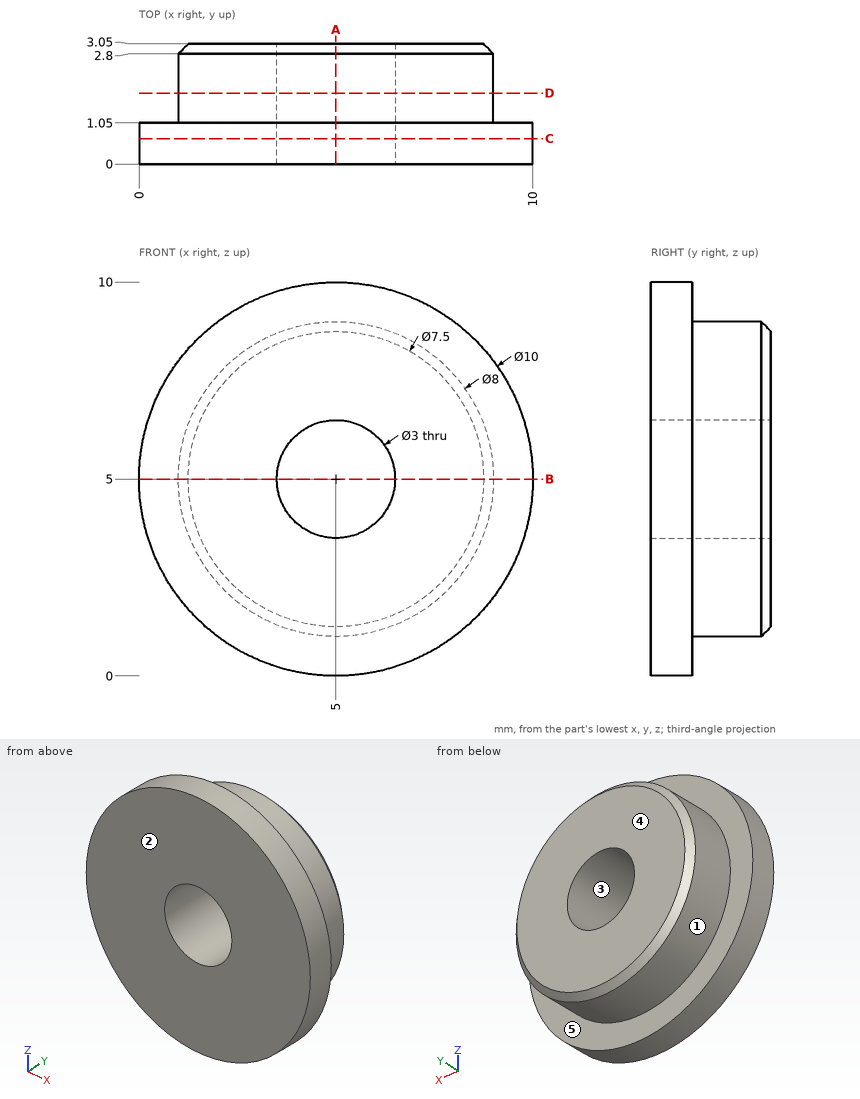
Geometry check sheet. Reference: drawing and pictorial views, mm from the part's lowest x, y, z. A direction names the side the tool comes from. Give positions to 0.01 mm unless a question says otherwise; leave off trailing zeros. Write each loop counter-clockwise with the first axis right and the second up, starting at its lowest first coordinate (ties: lowest second). Pieces come first, ordered by that corner, then holes.
Item 1: Cross-section at B-B (z = 5). Enter the section's corners in (x, y), and give its area (3 significant figures).
Item 2: Access from +Z, -Z, +X, -X, +Y, -Y to the whole of each face (thin tool, end or side, straight path). Record for the marked faces 4 and 5.
Item 3: Gauge pin test, flat end, axial feed: pin 1 (1.5 mm diameter, centred on y = 2.5, z = 5.5, fed in from -X). Record the tip position at first contact, or that the pin passes through.
Item 4: Scan lines: L1, parallel to X at y = 0.7, z = 5; L2, parallel to Z at x = 5, y = 1.9. Record each from-to range of solid material in increasing order.
Item 5: Cross-section at A-A (x = 5). Enter the section's corners in (y, z).
Item 6: Cross-section at D-D (y = 1.8). Enter the section's corners in (x, z).
Item 7: Draft check along Z on the marked faces 1, 2 and 3. Enter one of: released by +Z, released by -Z, zero draft, split by the parting line, or undercut.
Item 8: Cross-section at C-C (y = 0.65). Enter the section's corners in (x, z), and give its area (3 significant figures).
Report:
1. outline: (0, 0) - (3.5, 0) - (3.5, 3.05) - (1.25, 3.05) - (1, 2.8) - (1, 1.05) - (0, 1.05) - close; (6.5, 0) - (10, 0) - (10, 1.05) - (9, 1.05) - (9, 2.8) - (8.75, 3.05) - (6.5, 3.05) - close
1. area: 17.3 mm2
2. face 4: +Z, -Z, +X, -X, +Y
2. face 5: +Y
3. pin 1: stops at x = 1
4. L1: x = 0 to 3.5, 6.5 to 10
4. L2: z = 1 to 3.5, 6.5 to 9
5. outline: (0, 0) - (1.05, 0) - (1.05, 1) - (2.8, 1) - (3.05, 1.25) - (3.05, 3.5) - (0, 3.5) - close; (0, 6.5) - (3.05, 6.5) - (3.05, 8.75) - (2.8, 9) - (1.05, 9) - (1.05, 10) - (0, 10) - close
6. outline: circle Ø8 at (5, 5); hole circle Ø3 at (5, 5)
7. face 1: split by the parting line
7. face 2: zero draft
7. face 3: undercut
8. outline: circle Ø10 at (5, 5); hole circle Ø3 at (5, 5)
8. area: 71.5 mm2
